Design review of the part built by this model. Coordinates are the model's own, in mm. Coordinates: 2 decimals unless noted, no trailing zeros. Loops run counter-clockwise (first coordinate to the right, second up) from the corner with the lowest first, then second, coordinate; pieces in that order, holes last. Notation, with made-up numbers: M 16,-7.75 L 20,-7.75 A8 cw 20,-0.75 Z; hole C 68.5,13.25 d5. An arc over 180 degrees is marked long. Answer as a JSON object with one key per item and string values. Group by question number.
1. Consider section B-B (z = 18.5). State the section outline as (x, y) points, then the cut area to 3 significant figures.
2. Consider section A-A (y = 20.4). State the section outline as (x, z) points.
3. Consider section C-C (y = 44). State the section outline as (x, z) points, then the cut area to 3 significant figures.
4. Insertion check: pin 1 (2 mm diameter, centred on x = 41, y = 75.5, fed in from +Z); pin 2 (1.5 mm diameter, centred on x = 41.5, z = 15, fed in from +Y). Each pin has a flat end and moves straight along its axis. Give the tip position at first contact, or say it passes through.
5. To check wall thickness, follow probe 1 along Y at (x, z) = (41.05, 0); probe 2 along Y at (x, z) = (41.85, -12.5); probe 3 along X at (y, z) = (79, 23.5). State the ranges of each line that lie inside material, in increasing order.
Autodesk Inventor part; units mm, degrees
ref_plane "YZ Plane" through (0, 0, 0) normal (1, 0, 0) x (0, 1, 0)
ref_plane "XZ Plane" through (0, 0, 0) normal (0, 1, 0) x (-1, 0, 0)
ref_plane "XY Plane" through (0, 0, 0) normal (0, 0, 1) x (1, 0, 0)
sketch "스케치2" plane through (0, 0, 0) normal (0, 1, 0) x (-1, 0, 0)
  line L0 (0, 45) -> (38.9711, 22.5)
  line L1 (38.9711, 22.5) -> (38.9711, -22.5)
  line L2 (38.9711, -22.5) -> (0, -45)
  line L3 (0, -45) -> (-38.9711, -22.5)
  line L4 (-38.9711, -22.5) -> (-38.9711, 22.5)
  line L5 (-38.9711, 22.5) -> (0, 45)
  line L6 (0, 50.7735) -> (43.9711, 25.3868)
  line L7 (43.9711, 25.3868) -> (43.9711, -25.3868)
  line L8 (43.9711, -25.3868) -> (0, -50.7735)
  line L9 (0, -50.7735) -> (-43.9711, -25.3868)
  line L10 (-43.9711, -25.3868) -> (-43.9711, 25.3868)
  line L11 (-43.9711, 25.3868) -> (0, 50.7735)
  line L12 (-43.9711, 25.3868) -> (-38.9711, 22.5)
  line L13 (-38.9711, -22.5) -> (-43.9711, -25.3868)
  point P0 (0, 0)
  point P1 (0, 0)
  dimension "d0" = 45
  dimension "d1" = 5
extrude "돌출1" add sketch "스케치2" along normal blind 80 contours L4 L13 L10 L12
sketch "스케치3" plane through (38.9711, 0, -22.5) normal (-1, 0, 0) x (0, 0, 1)
  line L0 (0, 0) -> (45, 0) construction
  circle A0 centre (22.5, 20.4) radius 2.6
  point P0 (22.5, 0)
  point P1 (22.5, 0)
  dimension "d4" = 5.2
  dimension "d5" = 20.4
extrude "돌출2" cut sketch "스케치3" against normal through all
sketch "스케치4" plane through (0, 80, 0) normal (0, 1, 0) x (1, 0, 0)
  line L0 (38.9711, 22.5) -> (38.9711, -22.5) construction
  circle A0 centre (41.4711, 0) radius 2.5
  point P0 (0, 0)
  dimension "d8" = 5
extrude "돌출3" add sketch "스케치4" along normal blind 5
chamfer "모따기1" distance 1 angle 45 2 edges at (38.9711, 85, 0) (38.9711, 20.4, -2.6)
sketch "스케치5" plane through (43.9711, 0, 25.3868) normal (1, 0, 0) x (0, 0, -1)
  line L0 (50.7735, 0) -> (50.7735, 80) construction
  line L1 (25.3868, 80) -> (50.7735, 80) construction
  line L2 (0, 0) -> (0, 80) construction
  circle A0 centre (25.3868, 60) radius 2.6
  circle A1 centre (13.3868, 60) radius 2.6
  circle A2 centre (37.3868, 60) radius 2.6
  line L3 (0, 60) -> (50.7735, 60)
  point P0 (25.3868, 0)
  dimension "d11" = 20
  dimension "d12" = 0
  dimension "d13" = 0
  dimension "d14" = 0
  dimension "d15" = 12
  dimension "d16" = 12
  dimension "d17" = 5.2
  dimension "d18" = 5.2
  dimension "d19" = 5.2
properties part number "col_face"
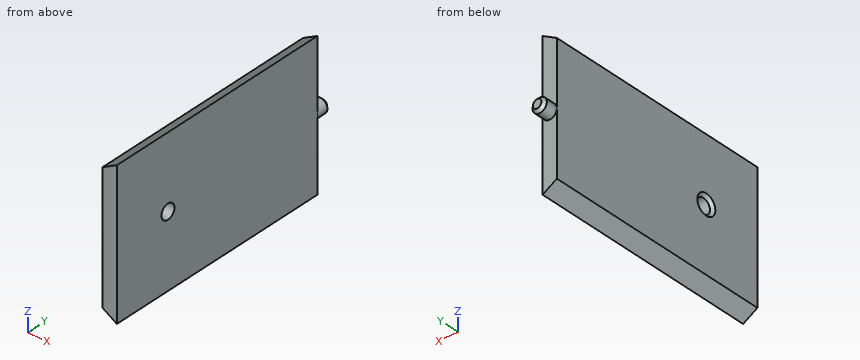
Findings below:
{
 "1": {"outline": "M 38.97,0 L 43.97,0 L 43.97,80 L 38.97,80 Z", "area": "400 mm^2"},
 "2": {"outline": "M 38.97,-22.5 L 43.97,-25.39 L 43.97,-2.6 L 39.97,-2.6 L 38.97,-3.6 Z; M 38.97,3.6 L 39.97,2.6 L 43.97,2.6 L 43.97,25.39 L 38.97,22.5 Z"},
 "3": {"outline": "M 38.97,-22.5 L 43.97,-25.39 L 43.97,25.39 L 38.97,22.5 Z", "area": "239 mm^2"},
 "4": {"pin 1": "stops at z = 24.25", "pin 2": "stops at y = 80"},
 "5": {"probe 1": "y = 0 to 17.8, 23 to 85", "probe 2": "y = 0 to 80", "probe 3": "x = 40.7 to 43.97"}
}
